Build history of the part. All positions in model axes, mm. A direction names the side the tool comes from. Give positions to 0.01 mm unless a question says otherwise; leave off trailing zeros. Order: outer loops, then holes, each group sorted by start corner. A loop starts at its lowest first (then second) coordinate and runs counter-clockwise, first axis right, second up. Notation, with made-up numbers: M 41.25,10.5 L 45.25,10.5 A24 ccw 45.25,24.5 Z; hole C -9.75,-31 d1. An arc over 180 degrees is marked long. Use CSV: the item, a comma, the result in double quotes. Start each with the question number.
Item 1: Pin check, flat tips, straight feed: P1, Ø5, axis at y = -0.83, z = -177.48, coming from the -X side; P2, Ø3, axis at y = 69.17, z = -177.48, coming from the +X side; P3, Ø3, axis at x = -18.5, y = 15, coming from the -Z side; P4, Ø4, axis at x = -20.5, y = 59, coming from the +Z side. Stop position of each tip, or through.
Item 2: Which spindle directions (+Z, -Z, +X, -X, +Y, -Y) get a long thin tool onto all of the face, cutting with end or side? Do faces 1 (the cylindrical face through (2.46, 69.91, -176.06)), 2 (the flat face through (-16, 34, -155.478)). Say none if no direction does.
Item 3: Band-saw the part on A-A on x = -17.5. Write the cut outline in (y, z).
Item 4: Two-plate mould, pull along X, no slides. Class faces 3 (the flat face through (0, 34, -175)), 4 (the cylindrical face through (2.46, 69.91, -166.06)), 5 (the cylindrical face through (-18.85, 12.53, -157.94)): pulls with the +X half, pulls with the -X half, needs draft (parallel to the pull), parting line crosses it, or undercut.
Item 5: Band-saw the part on C-C on x = -10. Write the cut outline in (y, z).
Item 6: Band-saw the part on B-B on y = 28. Write the cut outline in (x, z).
Item 7: Wall check: line 1 along X through (y, z) = (63, -182); line 2 along Z through (x, y) = (-25, 23.5); line 3 along X through (y, z) = (58.5, -154.5). Give the ranges that are in metal, low to high.
Autodesk Inventor part; units mm, degrees
ref_plane "YZ Plane" through (0, 0, 0) normal (1, 0, 0) x (0, 1, 0)
ref_plane "XZ Plane" through (0, 0, 0) normal (0, 1, 0) x (-1, 0, 0)
ref_plane "XY Plane" through (0, 0, 0) normal (0, 0, 1) x (1, 0, 0)
sketch "スケッチ1" plane through (0, 0, 0) normal (1, 0, 0) x (0, 1, 0)
  line L0 (-10.8312, -155.4782) -> (79.1688, -155.4782)
  line L1 (79.1688, -155.4782) -> (79.1688, -129.4782)
  line L2 (79.1688, -129.4782) -> (-10.8312, -129.4782)
  line L3 (-10.8312, -129.4782) -> (-10.8312, -155.4782)
  line L4 (-10.8312, -187.4782) -> (-10.8312, 372.5218)
  line L5 (79.1688, 372.5218) -> (79.1688, -187.4782)
  line L6 (-10.8312, -187.4782) -> (79.1688, -187.4782)
  line L7 (79.1688, -187.4782) -> (79.1688, -160.4782)
  line L8 (79.1688, -160.4782) -> (-10.8312, -160.4782)
  line L9 (-10.8312, -160.4782) -> (-10.8312, -187.4782)
  circle A0 centre (-0.8312, -167.4782) radius 1.6
  line L10 (-10.8312, -160.4782) -> (79.1688, -160.4782)
  line L11 (79.1688, -160.4782) -> (79.1688, -129.4782)
  line L12 (79.1688, -129.4782) -> (-10.8312, -129.4782)
  line L13 (-10.8312, -129.4782) -> (-10.8312, -160.4782)
  circle A1 centre (-0.8312, -167.4782) radius 1.6
  circle A2 centre (-0.8312, -177.4782) radius 1.6
  circle A3 centre (-0.8312, -177.4782) radius 1.6
  circle A4 centre (69.1688, -167.4782) radius 1.6
  circle A5 centre (69.1688, -167.4782) radius 1.6
  circle A6 centre (69.1688, -177.4782) radius 1.6
  circle A7 centre (69.1688, -177.4782) radius 1.6
  point P0 (0, 0)
  point P1 (-65.8312, -380.4782)
  dimension "d0" = 90
  dimension "d1" = 26
  dimension "d2" = 7
  dimension "d3" = 5
  dimension "d4" = 0
  dimension "d5" = 3.2
  dimension "d6" = 3.2
  dimension "d7" = 3.2
  dimension "d8" = 3.2
extrude "押し出し1" add sketch "スケッチ1" along normal blind 5
extrude "押し出し2" add sketch "スケッチ1" against normal blind 30 contours L0 L5 L8 L4
sketch "スケッチ2" plane through (0, -10.8312, -160.4782) normal (0, 0, -1) x (-1, 0, 0)
  line L0 (30, 90) -> (30, 0)
  line L1 (30, 45) -> (0, 45)
  line L2 (0, 0) -> (30, 0)
  line L3 (17.5, 0) -> (17.5, 90)
  line L4 (0, 90) -> (30, 90)
  circle A0 centre (17.5, 22.5) radius 1.6
  circle A1 centre (17.5, 67.5) radius 1.6
  point P0 (0, 10.8312)
  point P1 (15, 45)
  dimension "d13" = 12.5
  dimension "d14" = 3.2
  dimension "d15" = 3.2
  dimension "d16" = 22.5
  dimension "d17" = 22.5
hole "穴1" at (-17.5, 11.6688, -160.4782) at (-17.5, 56.6688, -160.4782) direction (0, 0, 1) diameter 3.2 end through all
fillet "フィレット1" radius 2 8 edges at (0, 34.1688, -160.4782) (-30, -10.8312, -157.9782) (-30, 79.1688, -157.9782) (0, 34.1688, -155.4782) (2.5, -10.8312, -187.4782) (2.5, 79.1688, -187.4782) (2.5, 79.1688, -129.4782) (2.5, -10.8312, -129.4782)
equation "\"d17\" = d16"
properties part number "dribl-v3-3DP-2" material "ABS プラスチック"
Model answer:
1,P1,"stops at x = 0"
1,P2,"passes through"
1,P3,"stops at z = -160.48"
1,P4,"stops at z = -155.48"
2,face 1,"+X, -X"
2,face 2,"+Z, -X, +Y, -Y"
3,outline,"M -10.83,-160.48 L 10.07,-160.48 L 10.07,-155.48 L -10.83,-155.48 Z; M 13.27,-160.48 L 55.07,-160.48 L 55.07,-155.48 L 13.27,-155.48 Z; M 58.27,-160.48 L 79.17,-160.48 L 79.17,-155.48 L 58.27,-155.48 Z"
4,face 3,"pulls with the -X half"
4,face 4,"needs draft"
4,face 5,"undercut"
5,outline,"M -10.83,-160.48 L 79.17,-160.48 L 79.17,-155.48 L -10.83,-155.48 Z"
6,outline,"M -30,-160.48 L -2,-160.48 A2 cw 0,-162.48 L 0,-187.48 L 5,-187.48 L 5,-129.48 L 0,-129.48 L 0,-153.48 A2 cw -2,-155.48 L -30,-155.48 Z"
7,line 1,"x = 0 to 5"
7,line 2,"z = -160.48 to -155.48"
7,line 3,"x = -0.28 to 5"
